Here's how the part is built. I have some questions about the finished solid (model axes, mm). Round coordinates to 2 decimals unless told otherwise and drop trailing zeros. Loops run counter-clockwise (first coordinate to the right, second up) from the corner with the lowest first, then second, coordinate; pieces in that order, holes last. Notation, with made-up numbers: M -35.5,10 L -3.5,10 A18 cw -3.5,32 Z; hole C -33,78.5 d9. An arc over 180 degrees is marked long. Answer as CSV lines item,"result".
```python
from build123d import *

# Parameters (mm, degrees)
SKETCH_F_W                   = 449
SKETCH_F_H                   = 79
SKETCH_F_R                   = 2.5
ESTRUSIONE_ESTRUSIONE1_DEPTH = 5
SKETCH1_R                    = 1.7
EXTRUDE1_DEPTH               = 6


with BuildPart() as part:
    # Sketch f → Estrusione-Estrusione1 (new body)
    with BuildSketch(Plane.XY):
        with Locations((224.5, 39.5)):
            Rectangle(SKETCH_F_W, SKETCH_F_H)
        with Locations((11.5, 67.5)):
            Circle(SKETCH_F_R, mode=Mode.SUBTRACT)
        with Locations((437.5, 67.5)):
            Circle(SKETCH_F_R, mode=Mode.SUBTRACT)
        with Locations((11.5, 11.5)):
            Circle(SKETCH_F_R, mode=Mode.SUBTRACT)
        with Locations((437.5, 11.5)):
            Circle(SKETCH_F_R, mode=Mode.SUBTRACT)
    extrude(amount=ESTRUSIONE_ESTRUSIONE1_DEPTH)

    # Sketch1 → Extrude1 (cut, through all)
    with BuildSketch(Plane(origin=(0, 0, 0), x_dir=(-1, 0, 0), z_dir=(0, 0, -1))):
        with Locations((-413.061242298, 39.505506417)):
            Circle(SKETCH1_R)
        with Locations((-357.061242298, 39.505506417)):
            Circle(SKETCH1_R)
        with BuildLine():
            Line((-364.0746338, 54.394920259), (-406.0746338, 54.394920259))
            ThreePointArc((-406.0746338, 54.394920259), (-408.903060925, 53.223347384), (-410.0746338, 50.394920259))
            Line((-410.0746338, 50.394920259), (-410.0746338, 28.394920259))
            ThreePointArc((-410.0746338, 28.394920259), (-408.903060925, 25.566493134), (-406.0746338, 24.394920259))
            Line((-406.0746338, 24.394920259), (-364.0746338, 24.394920259))
            ThreePointArc((-364.0746338, 24.394920259), (-361.246206675, 25.566493134), (-360.0746338, 28.394920259))
            Line((-360.0746338, 28.394920259), (-360.0746338, 50.394920259))
            ThreePointArc((-360.0746338, 50.394920259), (-361.246206675, 53.223347384), (-364.0746338, 54.394920259))
        make_face()
    extrude(amount=-EXTRUDE1_DEPTH, mode=Mode.SUBTRACT)


solid = part.part
```
1. I want a section at B-B, the plane z = 0.75. Please give me the cut outline in (x, y), and give its area (3 significant figures).
Evaluation:
outline,"M 0,0 L 449,0 L 449,79 L 0,79 Z; hole C 11.5,11.5 d5; hole C 11.5,67.5 d5; hole C 357.06,39.51 d3.4; hole M 360.07,28.39 A4 ccw 364.07,24.39 L 406.07,24.39 A4 ccw 410.07,28.39 L 410.07,50.39 A4 ccw 406.07,54.39 L 364.07,54.39 A4 ccw 360.07,50.39 Z; hole C 413.06,39.51 d3.4; hole C 437.5,11.5 d5; hole C 437.5,67.5 d5"
area,"33,900 mm²"
2. If I drill on line 1 (Y direction, x = 11.5, z = 1.75); line 2 (X direction, y = 31.5, z = 1.6); line 3 (Y direction, x = 395.5, z = 2.75), over which ranges is the centre line in solid material (lowest first)? Write a range as [from, to].
Evaluation:
line 1,"y = [0, 9], [14, 65], [70, 79]"
line 2,"x = [0, 360.07], [410.07, 449]"
line 3,"y = [0, 24.39], [54.39, 79]"
3. For P1, Ø1, axis at y = 41, z = 4, coming from the -X side, with a flat end and sliding along its axis, tell me the tip position at first contact or that it passes through.
Evaluation:
P1,"stops at x = 0"
4. I want a section at A-A, the plane x = 377.5. Please give me the cut outline in (y, z).
Evaluation:
outline,"M 0,0 L 24.39,0 L 24.39,5 L 0,5 Z; M 54.39,0 L 79,0 L 79,5 L 54.39,5 Z"
